Part model, mm, in its own coordinate system. Face numbers are marked on the shaded views. Give positions to 0.01 mm unless a question says otherwise; leave off trailing zeros. Loops run counter-clockwise (first coordinate to the right, second up) from the corner with the lowest first, then second, coordinate; pieces in that order, holes last. Notation, with made-up numbers: M -5,5 L 20,5 A20 ccw 20,14 Z; hole C 26,-29.75 d8. An arc over 180 degrees is marked long. Answer in a Markdown table with one row per item.
from build123d import *

# Parameters (mm, degrees)
F0_R     = 15
F0_R_2   = 10
F1_DEPTH = 25
F2_DEPTH = 50
F3_R     = 3.379899
F4_SIZE  = 2
F5_SIZE  = 1


with BuildPart() as f1:
    # F0 (on Front) → F1 (new body)
    with BuildSketch(Plane.XZ):
        with BuildLine():
            ThreePointArc((6.25, -29.341736), (23.318448, -18.874586), (30, 0))
            ThreePointArc((30, 0), (23.318448, 18.874586), (6.25, 29.341736))
            ThreePointArc((6.25, 29.341736), (-30, 0), (6.25, -29.341736))
        make_face()
        Circle(F0_R, mode=Mode.SUBTRACT)
        with BuildLine():
            ThreePointArc((6.25, 29.341736), (23.318448, 18.874586), (30, 0))
            ThreePointArc((30, 0), (23.318448, -18.874586), (6.25, -29.341736))
            Line((6.25, -29.341736), (63.645833, -17.116013))
            ThreePointArc((63.645833, -17.116013), (42.5, 0), (63.645833, 17.116013))
            Line((63.645833, 17.116013), (6.25, 29.341736))
        make_face()
        with BuildLine():
            ThreePointArc((77.5, 0), (73.602428, 11.010175), (63.645833, 17.116013))
            ThreePointArc((63.645833, 17.116013), (42.5, 0), (63.645833, -17.116013))
            ThreePointArc((63.645833, -17.116013), (73.602428, -11.010175), (77.5, 0))
        make_face()
        with Locations((60, 0)):
            Circle(F0_R_2, mode=Mode.SUBTRACT)
    extrude(amount=F1_DEPTH)

    # F0 (on Front) → F2 (join)
    with BuildSketch(Plane.XZ):
        with BuildLine():
            ThreePointArc((6.25, -29.341736), (23.318448, -18.874586), (30, 0))
            ThreePointArc((30, 0), (23.318448, 18.874586), (6.25, 29.341736))
            ThreePointArc((6.25, 29.341736), (-30, 0), (6.25, -29.341736))
        make_face()
        Circle(F0_R, mode=Mode.SUBTRACT)
    extrude(amount=F2_DEPTH)

    # F3
    f3_edges = [f1.edges().sort_by_distance(p)[0] for p in [
        (-30, 0, 0),
        (34.947917, 0, -23.228875),
        (77.5, 0, 0),
        (34.947917, 0, 23.228875),
    ]]
    fillet(f3_edges, radius=F3_R)

    # F4
    f4_edges = [f1.edges().sort_by_distance(p)[0] for p in [
        (-15, -50, 0),
        (50, -25, 0),
    ]]
    chamfer(f4_edges, length=F4_SIZE)

    # F5
    f5_edges = [f1.edges().sort_by_distance(p)[0] for p in [
        (-6.25, -50, 29.341736),
    ]]
    chamfer(f5_edges, length=F5_SIZE)


solid = f1.part
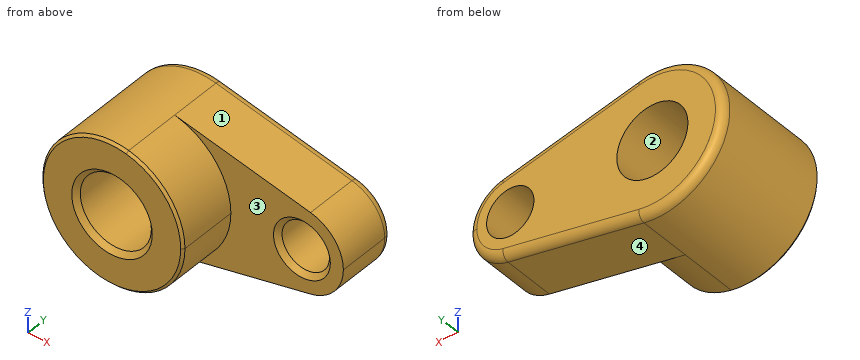
(1) Saw through at B-B (y = -44.5). Write the cut outline in (x, z).
Recorded:
| item | result |
|---|---|
| outline | M 6.25,-29.34 A30 ccw 30,0 A30 ccw 6.25,29.34 A30 ccw long Z; hole C 0,0 d30 |
(2) Saw through at C-C (z = -3). Give the number of separate pieces and of enclosed holes in the cut face, plus the area to 3 significant figures.
Recorded:
| item | result |
|---|---|
| separate pieces | 3 |
| enclosed holes | 0 |
| area | 2,210 mm^2 |
(3) Drill centre lines: line 1 along Z through (x, y) = (0, -10); line 2 along X through (y, z) = (-3, -2.5); line 3 along X through (y, z) = (-29, 0.5). Where is each one in solid material? Low to high.
Recorded:
| item | result |
|---|---|
| line 1 | z = -30 to -15, 15 to 30 |
| line 2 | x = -29.87 to -14.79, 14.79 to 50.32, 69.68 to 77.3 |
| line 3 | x = -30 to -14.99, 14.99 to 30 |
(4) Pull direction Z, two halves, no side cores. Call the marked faces 1, 2, 3 and 4: +Z half, -Z half, draft (parallel to the pull), parting line (faces both ways), or undercut.
Recorded:
| item | result |
|---|---|
| face 1 | +Z half |
| face 2 | undercut |
| face 3 | draft |
| face 4 | -Z half |
(5) Saw through at A-A (y = -12). Write the cut outline in (x, z), plus the area to 3 significant figures.
Recorded:
| item | result |
|---|---|
| outline | M 6.25,-29.34 L 63.65,-17.12 A17.5 ccw 63.65,17.12 L 6.25,29.34 A30 ccw long Z; hole C 0,0 d30; hole C 60,0 d20 |
| area | 3,790 mm^2 |
(6) Pin check, flat tips, straight feed: pin 1 Ø3 at (x, y) = (-10.5, -36) entering from +Z; pin 2 Ø4 at (y, z) = (-30.5, 8) entering from -X; pin 3 Ø1.5 at (y, z) = (-12.5, 12) entering from +X. Stop position of each tip, or through.
Recorded:
| item | result |
|---|---|
| pin 1 | stops at z = 28.62 |
| pin 2 | stops at x = -29.39 |
| pin 3 | stops at x = 73.4 |
